```python
from build123d import *

# Parameters (mm, degrees)
F0_W     = 25.4
F0_H     = 29.27313
F1_DEPTH = 25.4
F2_R     = 3.632204
F3_DEPTH = 30.226
F4_R     = 3.164391
F4_R_2   = 4.898125
F4_R_3   = 4.24451
F4_R_4   = 3.887819
F5_DEPTH = 25.401


with BuildPart() as f1:
    # F0 (on Front) → F1 (new body)
    with BuildSketch(Plane.XZ):
        with Locations((-0.414785, -0.999168)):
            Rectangle(F0_W, F0_H)
    extrude(amount=F1_DEPTH)

    # F2 (on face) → F3 (cut)
    with BuildSketch(Plane.XZ.offset(25.4)):
        with Locations((-8.4971, 5.941204)):
            Circle(F2_R)
    extrude(amount=-F3_DEPTH, mode=Mode.SUBTRACT)

    # F4 (on face) → F5 (cut, through all)
    with BuildSketch(Plane(origin=(0, 0, 0), x_dir=(-1, 0, 0), z_dir=(0, 1, 0))):
        with Locations((0, -0.979845)):
            Circle(F4_R)
        with Locations((7.981689, -7.926342)):
            Circle(F4_R_2)
        with Locations((-7.278915, -10.046526)):
            Circle(F4_R_3)
        with Locations((-5.619815, 5.608665)):
            Circle(F4_R_4)
    extrude(amount=-F5_DEPTH, mode=Mode.SUBTRACT)


solid = f1.part
```
Could you check a few things on this model? Use its own coordinates, in mm. Round coordinates to 2 decimals unless told otherwise and drop trailing zeros. Loops run counter-clockwise (first coordinate to the right, second up) from the corner with the lowest first, then second, coordinate; pieces in that order, holes last. Notation, with made-up numbers: (-3.75, -18.5) -> (10.25, -18.5) arc R23 cw to (10.25, 17.5) -> close; hole circle Ø5 at (25.25, 49). An arc over 180 degrees is marked (long way). Put each result on its own line as item: value.
Q1. For pin 1 Ø5.5 at (x, z) = (0, -0.98) entering from -Y; pin 2 Ø4 at (x, z) = (-2.5, -2) entering from +Y, each with a flat end and sliding along its axis, tell me the tip position at first contact or that it passes through.
Checks:
pin 1: through
pin 2: y = 0
Q2. I want a section at D-D on z = -2.25. Write out the boundary of the cut face in (x, y), and give its area (3 significant figures).
Checks:
outline: (-13.11, -25.4) -> (-2.9, -25.4) -> (-2.9, 0) -> (-13.11, 0) -> close; (2.9, -25.4) -> (12.29, -25.4) -> (12.29, 0) -> (2.9, 0) -> close
area: 498 mm2
Q3. I want a section at C-C on x = 8.5. Write out the boundary of the cut face in (y, z).
Checks:
outline: (-25.4, -15.64) -> (0, -15.64) -> (0, -14.11) -> (-25.4, -14.11) -> close; (-25.4, -5.98) -> (0, -5.98) -> (0, 3) -> (-25.4, 3) -> close; (-25.4, 8.22) -> (0, 8.22) -> (0, 13.64) -> (-25.4, 13.64) -> close
Q4. I want a section at B-B on z = -7.25. Write out the boundary of the cut face in (x, y), and give its area (3 significant figures).
Checks:
outline: (-13.11, -25.4) -> (-12.83, -25.4) -> (-12.83, 0) -> (-13.11, 0) -> close; (-3.13, -25.4) -> (4.09, -25.4) -> (4.09, 0) -> (-3.13, 0) -> close; (10.47, -25.4) -> (12.29, -25.4) -> (12.29, 0) -> (10.47, 0) -> close
area: 237 mm2
Q5. Thinking about a two-plate mould opening in Z: for faces 1 (the flat face through (-1, -13, -15.636)), 2 (the flat face through (-0.6, 0, 2.5)), 3 (the cylindrical face through (-6.92, -12.52, -12.71)), which applies, pulls with the +Z half, pulls with the -Z half, needs draft (parallel to the pull), parting line crosses it, or undercut?
Checks:
face 1: pulls with the -Z half
face 2: needs draft
face 3: undercut
Q6. Please list where these lines run through material, in increasing order: line 1 (X direction, y = -12, z = 8.25); line 2 (X direction, y = -9, z = 6); line 3 (Z direction, x = 4.25, y = -12.25). Write a range as from..to.
Checks:
line 1: -13.11..-11.3, -5.69..2.77, 8.47..12.29
line 2: -13.11..-12.13, -4.87..1.75, 9.49..12.29
line 3: -15.64..-13.02, -7.07..1.97, 9.25..13.64
Q7. I want a section at A-A on x = 0. Write out the boundary of the cut face in (y, z), and give its area (3 significant figures).
Checks:
outline: (-25.4, -15.64) -> (0, -15.64) -> (0, -4.14) -> (-25.4, -4.14) -> close; (-25.4, 2.18) -> (0, 2.18) -> (0, 13.64) -> (-25.4, 13.64) -> close
area: 583 mm2
